Check sheet for the drawn part. Datum: minimum x, y, z corner. Units: mm. A direction names the side the tool comes from. Round coordinates to 2 decimals unless told otherwise and drop trailing zeros. Write each loop counter-clockwise with the first axis right and the second up, starting at its lowest first coordinate (ties: lowest second). Pieces come first, ordered by that corner, then holes. Notation, with made-up numbers: (37, 75) - (83, 75) arc R26 cw to (83, 92) - close; hole circle Ø3 at (50.25, 41). An arc over 180 degrees is marked (long way). Write each question's results on one line, items separated by ' | '.
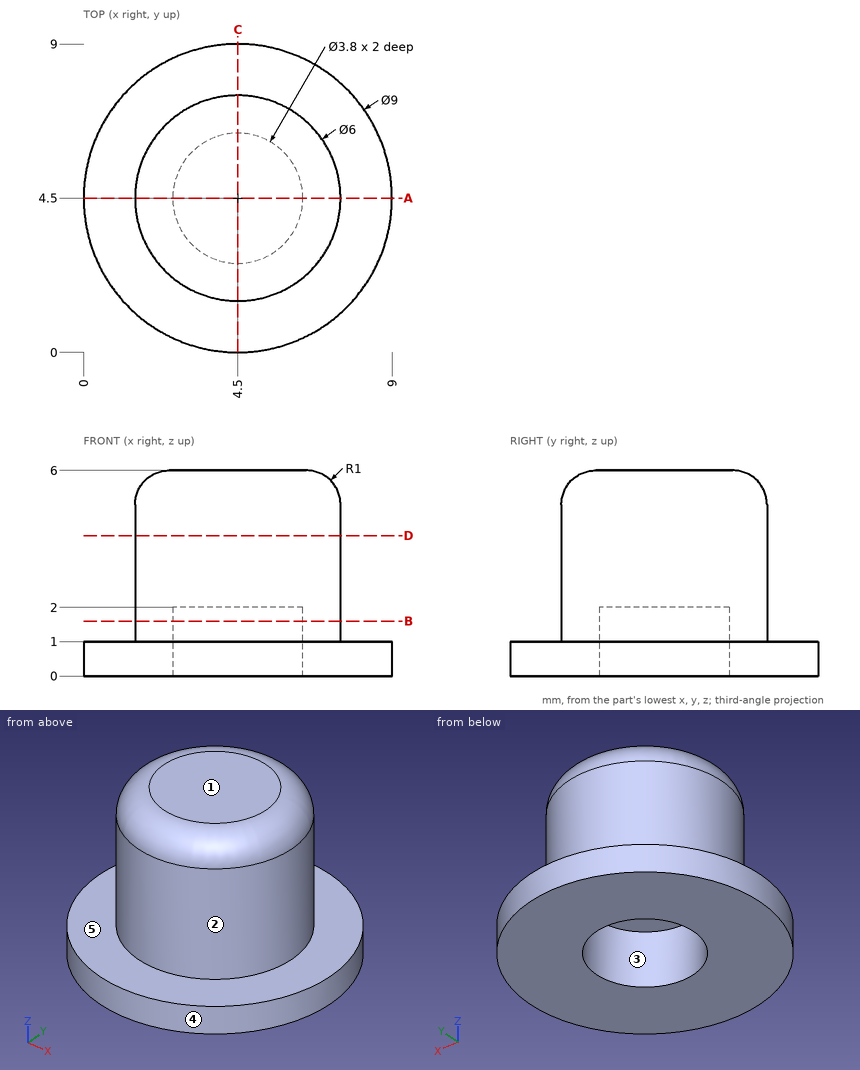
(1) Go/stop test with flat-tipped pins: pin 1 Ø1.5 at (x, z) = (7, 2) entering from -Y; pin 2 Ø1.5 at (y, z) = (3, 4.5) entering from +X; pin 3 Ø1 at (x, z) = (6.5, 0.5) entering from +Y. Record where each tip stops, or that it passes through.
Answer:
pin 1: y = 2.06 | pin 2: x = 7.4 | pin 3: y = 8.74
(2) Thickness scan on L1, parallel to Y at x = 4.5, z = 1.3; L2, parallel to Y at x = 4.5, z = 0.6; L3, parallel to Z at x = 2, y = 6.25. Record the ranges inside material, lowest first.
Answer:
L1: 1.5 to 2.6, 6.4 to 7.5 | L2: 0 to 2.6, 6.4 to 9 | L3: 0 to 1
(3) Section check D-D (z = 4.1). Record the cut outline in (x, y), plus the area to 3 significant figures.
Answer:
outline: circle Ø6 at (4.5, 4.5) | area: 28.3 mm2
(4) Set-up check for the marked faces 1 and 2: record each of +Z, -Z, +X, -X, +Y, -Y from which the full face is reachable in a straight line by a thin tool's end or side.
Answer:
face 1: +Z, +X, -X, +Y, -Y | face 2: +Z
(5) Section check A-A (y = 4.5). Record the cut outline in (x, z), plus the area to 3 significant figures.
Answer:
outline: (0, 0) - (2.6, 0) - (2.6, 2) - (6.4, 2) - (6.4, 0) - (9, 0) - (9, 1) - (7.5, 1) - (7.5, 5) arc R1 ccw to (6.5, 6) - (2.5, 6) arc R1 ccw to (1.5, 5) - (1.5, 1) - (0, 1) - close | area: 31.0 mm2
(6) Mould release check, pull along X, two halves, no side actions. Record for the marked faces 3, 4 and 5: released by +X, released by -X, zero draft, split by the parting line, or undercut.
Answer:
face 3: undercut | face 4: split by the parting line | face 5: zero draft
(7) Section check B-B (z = 1.6). Record the cut outline in (x, y), plus the area to 3 significant figures.
Answer:
outline: circle Ø6 at (4.5, 4.5); hole circle Ø3.8 at (4.5, 4.5) | area: 16.9 mm2
